from build123d import *

# Parameters (mm, degrees)
F0_R     = 3.5
F0_R_2   = 3
F1_DEPTH = 1
F2_R     = 5
F2_R_2   = 3.5
F2_R_3   = 3
F3_DEPTH = 8
F4_R     = 2.5
F4_R_2   = 2
F5_DEPTH = 1.4
F7_DEPTH = 5


# Not quite as in the source:
# - a fillet or chamfer that OpenCascade refuses, or shapes differently, is made with other operations: its cross-section is extruded or revolved along the edge and cut away or added


with BuildPart() as f1:
    # F0 (on Top) → F1 (new body)
    with BuildSketch(Plane.XY):
        Circle(F0_R)
        Circle(F0_R_2, mode=Mode.SUBTRACT)
    extrude(amount=F1_DEPTH)

    # F2 (on face) → F3 (join)
    with BuildSketch(Plane.XY.offset(1)):
        Circle(F2_R)
        Circle(F2_R_2, mode=Mode.SUBTRACT)
        Circle(F2_R_2)
        Circle(F2_R_3, mode=Mode.SUBTRACT)
        Circle(F2_R_3)
    extrude(amount=F3_DEPTH)

    # F4 (on face) → F5 (join)
    with BuildSketch(Plane.XY.offset(9)):
        Circle(F4_R)
        Circle(F4_R_2, mode=Mode.SUBTRACT)
    extrude(amount=F5_DEPTH)

    # F6: fillet of radius 2 on 2 edges, made by hand

    # F6_s1 → F6_t2 (revolve, cut)
    with BuildSketch(Plane.XZ):
        with BuildLine():
            ThreePointArc((5, 7), (4.4142135624, 8.4142135624), (3, 9))
            Line((3, 9), (5, 9))
            Line((5, 9), (5, 7))
        make_face()
    revolve(axis=Axis((0, 0, 9), (0, 0, 1)), mode=Mode.SUBTRACT)

    # F6_s3 → F6_t4 (revolve, cut)
    with BuildSketch(Plane.XZ):
        with BuildLine():
            ThreePointArc((5, 2.9364916731), (4.5811388301, 1.7117468017), (3.5, 1))
            Line((3.5, 1), (5, 1))
            Line((5, 1), (5, 2.9364916731))
        make_face()
    revolve(axis=Axis((0, 0, 1), (0, 0, 1)), mode=Mode.SUBTRACT)

    # F7 (cut): a face of the model
    f7_faces = [f1.faces().sort_by_distance(p)[0] for p in [
        (0, 0, 1),
    ]]
    extrude(f7_faces, amount=-F7_DEPTH, mode=Mode.SUBTRACT)


solid = f1.part
Model file for the job. Use its own axes, mm. A direction names the side the tool comes from. Coordinates: 2 decimals unless noted, no trailing zeros. Write each loop counter-clockwise with the first axis right and the second up, starting at its lowest first coordinate (ties: lowest second). Pieces come first, ordered by that corner, then holes. Notation, with made-up numbers: (64.5, 71.5) -> (110.5, 71.5) arc R17 ccw to (110.5, 81.5) -> close; hole circle Ø8 at (-34.75, 48.5). An arc over 180 degrees is marked (long way). One line per item, written item: value. Start each with the question number.
1) Slice it at C-C on z = 9.75. Write the cut outline in (x, y).
2) Probe probe 1 along Y at (x, z) = (0, 4.7); probe 2 along Y at (x, z) = (0, 9.5); probe 3 along X at (y, z) = (-1.5, 10). List the from-to ranges inside material, lowest first.
3) Slice it at A-A on y = 0. Write the cut outline in (x, z).
4) Which spindle directions (+Z, -Z, +X, -X, +Y, -Y) get a long thin tool onto all of the face, cutting with end or side? Do faces 1 (the face through (-1.08, -4.88, 4.94)), 2 (the face through (-3, 0, 3)), 3 (the face through (-0.54, -2.44, 9.69)). Say none if no direction does.
5) Pull direction X, two halves, no side cores. Call faces 4 (the face through (0, -2, 10)), 5 (the face through (3.233, -1.341, 0.493)), 6 (the face through (-1, 2, 10.4)): +X half, -X half, draft (parallel to the pull), parting line (faces both ways), or undercut.
6) Slice it at D-D on z = 6.75. Write the cut outline in (x, y), then the cut area to 3 significant figures.
7) Flat gauge pins, fed straight in: pin 1 Ø4.5 at (x, y) = (-0.5, -1) entering from +Z; pin 2 Ø3.5 at (x, y) = (0, 0) entering from +Z; pin 3 Ø1 at (x, y) = (3, 3) entering from +Z; pin 4 Ø2 at (y, z) = (-3.5, 8.5) entering from -X. Where does each tip first touch, or does it go through?
Answers follow:
1. outline: circle Ø5 at (0, 0); hole circle Ø4 at (0, 0)
2. probe 1: -5 to -3, 3 to 5
2. probe 2: -2.5 to -2, 2 to 2.5
2. probe 3: -2 to -1.32, 1.32 to 2
3. outline: (-5, 2.94) arc R2 ccw to (-3.5, 1) -> (-3.5, 0) -> (-3, 0) -> (-3, 6) -> (3, 6) -> (3, 0) -> (3.5, 0) -> (3.5, 1) arc R2 ccw to (5, 2.94) -> (5, 7) arc R2 ccw to (3, 9) -> (2.5, 9) -> (2.5, 10.4) -> (2, 10.4) -> (2, 9) -> (-2, 9) -> (-2, 10.4) -> (-2.5, 10.4) -> (-2.5, 9) -> (-3, 9) arc R2 ccw to (-5, 7) -> close
4. face 1: +Z, -Z
4. face 2: -Z
4. face 3: +Z
5. face 4: undercut
5. face 5: parting line
5. face 6: draft
6. outline: circle Ø10 at (0, 0)
6. area: 78.5 mm2
7. pin 1: z = 10.4
7. pin 2: z = 9
7. pin 3: z = 8.86
7. pin 4: x = -3.95
